from build123d import *

# Parameters (mm, degrees)
AUFSATZ_LINEAR_AUSTRAGEN1_DEPTH = 35
SCHNITT_LINEAR_AUSTRAGEN1_DEPTH = 9


with BuildPart() as part:
    # Skizze1 → Aufsatz-Linear austragen1 (new body)
    with BuildSketch(Plane.XY):
        with BuildLine():
            add(Edge.make_bspline(
                [(4.5, 9.75), (1.282885482, 4.095735731), (3.75, -1.036897294)],
                knots=[0, 0, 0, 1, 1, 1], degree=2))
            Line((3.75, -1.036897294), (5.25, -1.036897294))
            add(Edge.make_bspline(
                [(6, 9.75), (2.782885482, 4.095735731), (5.25, -1.036897294)],
                knots=[0, 0, 0, 1, 1, 1], degree=2))
            Line((6, 9.75), (6, 13.75))
            Line((6, 13.75), (-7, 13.75))
            Line((-7, 13.75), (-7, 10.25))
            Line((-7, 10.25), (-5.5, 10.25))
            Line((-5.5, 10.25), (-5.5, 12.25))
            Line((-5.5, 12.25), (-1, 12.25))
            Line((-1, 12.25), (-1, -12.25))
            Line((-1, -12.25), (-5.5, -12.25))
            Line((-5.5, -12.25), (-5.5, -10.25))
            Line((-5.5, -10.25), (-7, -10.25))
            Line((-7, -10.25), (-7, -13.75))
            Line((-7, -13.75), (1, -13.75))
            Line((1, -13.75), (1, 12.25))
            Line((1, 12.25), (4.5, 12.25))
            Line((4.5, 12.25), (4.5, 9.75))
        make_face()
    extrude(amount=AUFSATZ_LINEAR_AUSTRAGEN1_DEPTH)

    # Skizze3 → Schnitt-Linear austragen1 (cut)
    with BuildSketch(Plane.XY.offset(35)):
        Polygon((-1, 12.25), (-1, 13.75), (-7, 13.75), (-7, 10.25), (-5.5, 10.25), (-5.5, 12.25), align=None)
    extrude(amount=-SCHNITT_LINEAR_AUSTRAGEN1_DEPTH, mode=Mode.SUBTRACT)


solid = part.part
For this review, take the finished solid that the model builds, in its own axes (mm). A direction names the side the tool comes from. Round coordinates to 2 decimals unless told otherwise and drop trailing zeros. Loops run counter-clockwise (first coordinate to the right, second up) from the corner with the lowest first, then second, coordinate; pieces in that order, holes last. Notation, with made-up numbers: (23.5, 13.5) - (66.5, 13.5) arc R19 cw to (66.5, 33.5) - close; hole circle Ø3 at (0, 79.5). An arc over 180 degrees is marked (long way). Use one line per item in the form item = value.
1) We need section B-B on y = -9.5. Write out the cut boundary in (x, z), then the cut area to 3 significant figures.
Solutions:
outline = (-1, 0) - (1, 0) - (1, 35) - (-1, 35) - close
area = 70.0 mm2
2) Wall thickness on probe 1 along X at (y, z) = (11.75, 16); probe 2 along X at (y, z) = (-11, 33); probe 3 along Y at (x, z) = (-6.5, 4): over which ranges is each line inside the solid? List them lowest first.
Solutions:
probe_1 = -7 to -5.5, -1 to 1, 4.5 to 6
probe_2 = -7 to -5.5, -1 to 1
probe_3 = -13.75 to -10.25, 10.25 to 13.75
3) Mouldability with a two-part tool opening along X and no side actions: class faces 6 (the face through (1, -1, 17)), 7 (the face through (-5, 13, 26)), 8 (the face through (-7, 12, 13)) as pulls with the +X half, pulls with the -X half, needs draft (parallel to the pull), parting line crosses it, or undercut.
Solutions:
face_6 = undercut
face_7 = needs draft
face_8 = pulls with the -X half
4) Tool access review of faces 1 (the face through (4, -1.037, 17)), 2 (the face through (-7, -12, 17)), 3 (the face through (0, 1, 35)), 4 (the face through (3, 12.25, 17)), 5 (the face through (-6, -10.25, 17)): name each direction out of +Z, -Z, +X, -X, +Y, -Y from which nothing blocks a thin tool from reaching the whole face with its end or side.
Solutions:
face_1 = +Z, -Z, +X, -Y
face_2 = +Z, -Z, -X, +Y, -Y
face_3 = +Z, +X, -X, +Y, -Y
face_4 = +Z, -Z
face_5 = +Z, -Z, -X
5) Clearance check with flat-ended pins moving along their axes: P1, Ø1.6, axis at y = -11.5, z = 20.5, coming from the +X side; P2, Ø1.8, axis at x = -4.5, y = 12.5, coming from the +Z side; P3, Ø3, axis at x = 1, y = 6, coming from the -Z side; P4, Ø3, axis at y = -2.5, z = 29, coming from the +X side. State where each tip first meets the part, or that it passes through.
Solutions:
P1 = 1
P2 = 26
P3 = 0
P4 = 5.25
6) We need section A-A on x = -2.75. Write out the cut boundary in (y, z), then the cut area to 3 significant figures.
Solutions:
outline = (-13.75, 0) - (-12.25, 0) - (-12.25, 35) - (-13.75, 35) - close; (12.25, 0) - (13.75, 0) - (13.75, 26) - (12.25, 26) - close
area = 91.5 mm2
7) We need section C-C on x = 2. Write out the cut boundary in (y, z).
Solutions:
outline = (12.25, 0) - (13.75, 0) - (13.75, 35) - (12.25, 35) - close
